```python
from build123d import *

# Parameters (mm, degrees)
HOLE001_D           = 3.2
HOLE001_DEPTH       = 10
HOLE001_CBORE_D     = 6.5
HOLE001_CBORE_DEPTH = 3.1
HOLE001_TIPS_R      = 1.6


with BuildPart() as part:
    # Sketch060 → Revolution001 (revolve)
    with BuildSketch(Plane.XY):
        Polygon((0, 0), (-5, 0), (-5, -5), (-10, -9.195498), (-10, -10), (0, -10), align=None)
    revolve(axis=Axis((0, 0, 0), (0, 1, 0)))

    # Hole001
    with Locations(Plane.XZ.offset(10)):
        with Locations((0, 0)):
            CounterBoreHole(HOLE001_D / 2, HOLE001_CBORE_D / 2, HOLE001_CBORE_DEPTH, depth=HOLE001_DEPTH)

    # Hole001 tips → Hole001 tip 1 section 0
    with BuildSketch(Plane.XZ, mode=Mode.PRIVATE) as hole001_tip_1_s0:
        Circle(HOLE001_TIPS_R)
    loft([hole001_tip_1_s0.sketch, Vertex(0, 0.961377, 0)], mode=Mode.SUBTRACT)


with BuildPart() as part_1:
    # Body008 placement: moved
    add(part.part.moved(Location((0, -172, -53.5))))


solid = part_1.part
```
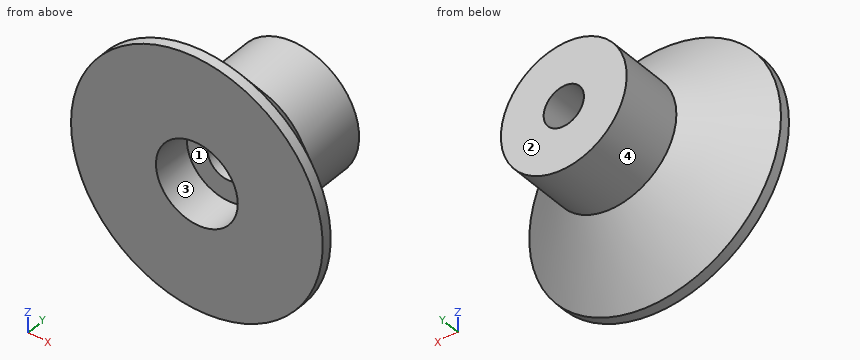
Check sheet for the modelled part. Datum: model origin and axes. Units: mm. Face numbers are marked on the shaded views. Coordinates: 2 decimals unless noted, no trailing zeros. Loops run counter-clockwise (first coordinate to the right, second up) from the corner with the lowest first, then second, coordinate; pieces in that order, holes last.
1) Sectioned sample at A-A (x = 0). Record the boundary of the cut face in (y, z).
2) Gauge pin test, flat ends, axial feed: pin 1 (3 mm diameter, centred on x = -0.5, z = -53, fed in from -Y); pin 2 (3 mm diameter, centred on y = -177.5, z = -51, fed in from -X); pin 3 (5 mm diameter, centred on x = -6.5, z = -58, fed in from +Y). Record the tip position at first contact, or that the pin passes through.
3) Sectioned sample at C-C (y = -176.5). Record the boundary of the cut face in (x, z), and give its area (3 significant figures).
4) Release check for a two-part mould opening along Z. For the marked faces 1, 2, 3 and 4 record: released by +Z, released by -Z, zero draft, split by the parting line, or undercut.
5) Sectioned sample at B-B (z = -53.5). Record the boundary of the cut face in (x, y).
6) Material ranges on probe 1 along Z at (x, y) = (0, -175.5); probe 2 along Z at (x, y) = (0, -180.15); probe 3 along Y at (x, z) = (1, -46.5), recorded low to high.
7) Sectioned sample at D-D (y = -180.5). Record the boundary of the cut face in (x, z), and give its area (3 significant figures).
Check sheet entries:
1. outline: (-182, -63.5) - (-181.2, -63.5) - (-177, -58.5) - (-172, -58.5) - (-172, -55.1) - (-178.9, -55.1) - (-178.9, -56.75) - (-182, -56.75) - close; (-182, -50.25) - (-178.9, -50.25) - (-178.9, -51.9) - (-172, -51.9) - (-172, -48.5) - (-177, -48.5) - (-181.2, -43.5) - (-182, -43.5) - close
2. pin 1: stops at y = -178.9
2. pin 2: stops at x = -7.01
2. pin 3: stops at y = -177.34
3. outline: circle Ø10 at (0, -53.5); hole circle Ø3.2 at (0, -53.5)
3. area: 70.5 mm2
4. face 1: undercut
4. face 2: zero draft
4. face 3: undercut
4. face 4: split by the parting line
5. outline: (-10, -182) - (-3.25, -182) - (-3.25, -178.9) - (-1.6, -178.9) - (-1.6, -172) - (-5, -172) - (-5, -177) - (-10, -181.2) - close; (1.6, -178.9) - (3.25, -178.9) - (3.25, -182) - (10, -182) - (10, -181.2) - (5, -177) - (5, -172) - (1.6, -172) - close
6. probe 1: z = -58.5 to -55.1, -51.9 to -48.5
6. probe 2: z = -62.25 to -56.75, -50.25 to -44.75
6. probe 3: y = -182 to -178.74
7. outline: circle Ø18.34 at (0, -53.5); hole circle Ø6.5 at (0, -53.5)
7. area: 231 mm2
